Here's how the part is built. I have some questions about the finished solid (model axes, mm). A direction names the side the tool comes from. Coordinates: 2 decimals unless noted, no trailing zeros. Write each loop counter-clockwise with the first axis right and the second up, starting at its lowest first coordinate (ties: lowest second). Pieces come first, ordered by that corner, then holes.
```python
from build123d import *

# Parameters (mm, degrees)
F2_R     = 10.5
F3_DEPTH = 66.001
F4_R     = 1
F5_DEPTH = 4


with BuildPart() as f1:
    # F0 (on Front) → F1 (revolve)
    with BuildSketch(Plane.XZ):
        Polygon((-36, 0), (0, 0), (0, 66), (-32, 66), (-32, 56), (-15, 56), (-15, 12), (-36, 12), align=None)
    revolve(axis=Axis((0, 0, 33), (0, 0, -1)))

    # F2 (on face) → F3 (cut, through all)
    with BuildSketch(Plane.XY.offset(66)):
        Circle(F2_R)
    extrude(amount=-F3_DEPTH, mode=Mode.SUBTRACT)

    # F4 (on face) → F5 (join)
    with BuildSketch(Plane.XY.offset(66)):
        with Locations((-29, 0)):
            Circle(F4_R)
        with Locations((29, 0)):
            Circle(F4_R)
    extrude(amount=F5_DEPTH)


solid = f1.part
```
1) On a 3-axis mill with a long thin cutter (end or side, diameter ignored), from which of +Z, -Z, +X, -X, +Y, -Y can I reach the whole of each face in a straight line? I mean faces 1 (the face through (14.985, 0.66, 33.692)), 2 (the face through (30, 0, 68)), 3 (the face through (10, 3.2, 33.5)). Say none if no direction works.
Values follow:
face 1: none
face 2: +Z
face 3: +Z, -Z
2) Will these pins go through, and if not, where does the flat tip stop? pin 1 (1 mm diameter, centred on x = 10.5, z = 35, fed in from +Y); pin 2 (12 mm diameter, centred on y = -17.5, z = 23.5, fed in from +X); pin 3 (8 mm diameter, centred on x = 12.5, y = 13, fed in from -Z); pin 4 (5 mm diameter, centred on x = 19.5, y = -19.5, fed in from +Z).
Values follow:
pin 1: stops at y = 11.18
pin 2: stops at x = 9.63
pin 3: stops at z = 0
pin 4: stops at z = 66
3) We'd pull the mould along Z, two halves only. Please class faces 4 (the face through (-14, -7, 56)), 5 (the face through (4.686, 35.694, 5.916)), 6 (the face through (29, 0, 70)): pulls with the +Z half, pulls with the -Z half, needs draft (parallel to the pull), parting line crosses it, or undercut.
Values follow:
face 4: undercut
face 5: needs draft
face 6: pulls with the +Z half
4) Imagine slicing it at C-C on z = 33. Please give me the cut outline in (x, y).
Values follow:
outline: circle Ø30 at (0, 0); hole circle Ø21 at (0, 0)
5) Imagine slicing it at B-B on x = 0. Please give me the cut outline in (y, z), then the cut area to 3 significant figures.
Values follow:
outline: (-36, 0) - (-10.5, 0) - (-10.5, 66) - (-32, 66) - (-32, 56) - (-15, 56) - (-15, 12) - (-36, 12) - close; (10.5, 0) - (36, 0) - (36, 12) - (15, 12) - (15, 56) - (32, 56) - (32, 66) - (10.5, 66) - close
area: 1,440 mm2
6) I need wall thicknesses on probe 1 along Z at (x, y) = (-14, 17.5); probe 2 along Y at (x, z) = (0, 19.5); probe 3 along X at (y, z) = (-4, 54). Which ranges of each line are inside material? Lowest first, please.
Values follow:
probe 1: z = 0 to 12, 56 to 66
probe 2: y = -15 to -10.5, 10.5 to 15
probe 3: x = -14.46 to -9.71, 9.71 to 14.46
7) Imagine slicing it at A-A on y = 0. Please give me the cut outline in (x, z), then the cut area to 3 significant figures.
Values follow:
outline: (-36, 0) - (-10.5, 0) - (-10.5, 66) - (-28, 66) - (-28, 70) - (-30, 70) - (-30, 66) - (-32, 66) - (-32, 56) - (-15, 56) - (-15, 12) - (-36, 12) - close; (10.5, 0) - (36, 0) - (36, 12) - (15, 12) - (15, 56) - (32, 56) - (32, 66) - (30, 66) - (30, 70) - (28, 70) - (28, 66) - (10.5, 66) - close
area: 1,450 mm2
8) Imagine slicing it at D-D on y = 21. Please give me the cut outline in (x, z), then the cut area to 3 significant figures.
Values follow:
outline: (-29.24, 0) - (29.24, 0) - (29.24, 12) - (-29.24, 12) - close; (-24.15, 56) - (24.15, 56) - (24.15, 66) - (-24.15, 66) - close
area: 1,180 mm2
